The listing builds one solid part. Answer for the finished solid, in the listing's coordinates (mm). A direction names the side the tool comes from. Coordinates: 2 decimals unless noted, no trailing zeros. Order: outer loops, then holes, each group sorted by start corner. A loop starts at its lowest first (then second) coordinate and runs counter-clockwise, first axis right, second up. Notation, with made-up numbers: (26, 82.5) - (55, 82.5) arc R16 cw to (55, 106.5) - close; hole circle Ø3 at (-4.75, 25.25). An arc over 180 degrees is marked (long way). One line per item, written item: value. Start each with the question number.
```python
from build123d import *

# Parameters (mm, degrees)
SKETCH1_W           = 10
SKETCH1_H           = 10
SKETCH1_R           = 1.6
BOSS_EXTRUDE1_DEPTH = 0.5
SKETCH4_W           = 10
SKETCH4_H           = 10
SKETCH4_W_2         = 9
SKETCH4_H_2         = 9
BOSS_EXTRUDE2_DEPTH = 9
SKETCH5_W           = 10
SKETCH5_H           = 10
SKETCH5_R           = 3
BOSS_EXTRUDE3_DEPTH = 0.5
SKETCH6_R           = 3
CUT_EXTRUDE1_DEPTH  = 0.5
SKETCH7_R           = 3
CUT_EXTRUDE2_DEPTH  = 0.5
SKETCH8_R           = 1.6
CUT_EXTRUDE3_DEPTH  = 0.5
SKETCH9_R           = 1.6
CUT_EXTRUDE4_DEPTH  = 0.5
FILLET5_R           = 0.5


with BuildPart() as part:
    # Sketch1 → Boss-Extrude1 (new body)
    with BuildSketch(Plane(origin=(0, 0, 0), x_dir=(1, 0, 0), z_dir=(0, 1, 0))):
        with Locations((5, 5)):
            Rectangle(SKETCH1_W, SKETCH1_H)
        with Locations(Location((5, 5, 0), (0, 0, 270))):
            Circle(SKETCH1_R, mode=Mode.SUBTRACT)
    extrude(amount=BOSS_EXTRUDE1_DEPTH)

    # Sketch4 → Boss-Extrude2 (add)
    with BuildSketch(Plane(origin=(0, 0.5, 0), x_dir=(1, 0, 0), z_dir=(0, 1, 0))):
        with Locations((5, 5)):
            Rectangle(SKETCH4_W, SKETCH4_H)
        with Locations((5, 5)):
            Rectangle(SKETCH4_W_2, SKETCH4_H_2, mode=Mode.SUBTRACT)
    extrude(amount=BOSS_EXTRUDE2_DEPTH)

    # Sketch5 → Boss-Extrude3 (add)
    with BuildSketch(Plane(origin=(0, 9.5, 0), x_dir=(1, 0, 0), z_dir=(0, 1, 0))):
        with Locations((5, 5)):
            Rectangle(SKETCH5_W, SKETCH5_H)
        with Locations(Location((5, 5, 0), (0, 0, 270))):
            Circle(SKETCH5_R, mode=Mode.SUBTRACT)
    extrude(amount=BOSS_EXTRUDE3_DEPTH)

    # Sketch6 → Cut-Extrude1 (cut)
    with BuildSketch(Plane(origin=(10, 0, 0), x_dir=(0, 0, -1), z_dir=(1, 0, 0))):
        with Locations((5, 5)):
            Circle(SKETCH6_R)
    extrude(amount=-CUT_EXTRUDE1_DEPTH, mode=Mode.SUBTRACT)

    # Sketch7 → Cut-Extrude2 (cut)
    with BuildSketch(Plane.XY):
        with Locations((5, 5)):
            Circle(SKETCH7_R)
    extrude(amount=-CUT_EXTRUDE2_DEPTH, mode=Mode.SUBTRACT)

    # Sketch8 → Cut-Extrude3 (cut)
    with BuildSketch(Plane.ZY):
        with Locations((-5, 5)):
            Circle(SKETCH8_R)
    extrude(amount=-CUT_EXTRUDE3_DEPTH, mode=Mode.SUBTRACT)

    # Sketch9 → Cut-Extrude4 (cut)
    with BuildSketch(Plane(origin=(0, 0, -10), x_dir=(-1, 0, 0), z_dir=(0, 0, -1))):
        with Locations((-5, 5)):
            Circle(SKETCH9_R)
    extrude(amount=-CUT_EXTRUDE4_DEPTH, mode=Mode.SUBTRACT)

    # Fillet5
    fillet5_edges = [part.edges().sort_by_distance(p)[0] for p in [
        (0, 10, -5),
        (5, 10, 0),
        (10, 10, -5),
        (5, 10, -10),
        (5, 0, -10),
        (10, 0, -5),
        (5, 0, 0),
        (0, 0, -5),
        (0, 5, -10),
        (10, 5, -10),
        (10, 5, 0),
        (0, 5, 0),
    ]]
    fillet(fillet5_edges, radius=FILLET5_R)


solid = part.part
```
(1) The part is cut by section C-C on x = 6. Determine the outline of the cut face in (y, z).
(2) The part is cut by section A-A on y = 1.25. Determine the outline of the cut face in (x, z), plus the area to 3 significant figures.
(3) For a pull along Z with two mould halves and no side action, classify faces 1 (the face through (2.338, 9.746, -3.616)), 2 (the face through (5, 0, -3)), 3 (the face through (5, 7, -10)) as pulls with the +Z half, pulls with the -Z half, needs draft (parallel to the pull), parting line crosses it, or undercut.
(4) Consider probe 1 along Y at (x, z) = (7.5, -7.75); probe 2 along Z at (x, y) = (7.75, 7). Determine where each line is inside the solid, lowest interval first.
(5) The part is cut by section D-D on y = 6.75. Determine the outline of the cut face in (x, z).
(6) The part is cut by section B-B on z = -5. Determine the outline of the cut face in (x, y), plus the area to 3 significant figures.
(7) Flat-ended cylindrical pins translate along their axes: pin 1 Ø1.9 at (y, z) = (5, -5) entering from -X; pin 2 Ø4.5 at (y, z) = (5.5, -7) entering from +X; pin 3 Ø4 at (x, z) = (5, -5) entering from +Y. Find the tip coordinate at first contact, or state that the pin passes through.
(8) For faces 4 (the face through (4.35, 2.07, -0.25)), 5 (the face through (9.75, 2.07, -4.35)), 6 (the face through (5, 7, -9.5)), determine the directions among +Z, -Z, +X, -X, +Y, -Y from which every point of the face is accessible in a straight line to the end or side of a thin tool.
Completed:
1. outline: (0, -9.5) arc R0.5 ccw to (0.5, -10) - (3.75, -10) - (3.75, -9.5) - (0.5, -9.5) - (0.5, -6.25) - (0, -6.25) - close; (0, -3.75) - (0.5, -3.75) - (0.5, -0.5) - (2.17, -0.5) - (2.17, 0) - (0.5, 0) arc R0.5 ccw to (0, -0.5) - close; (6.25, -10) - (9.5, -10) arc R0.5 ccw to (10, -9.5) - (10, -7.83) - (9.5, -7.83) - (9.5, -9.5) - (6.25, -9.5) - close; (7.83, -0.5) - (9.5, -0.5) - (9.5, -2.17) - (10, -2.17) - (10, -0.5) arc R0.5 ccw to (9.5, 0) - (7.83, 0) - close
2. outline: (0, -9.5) arc R0.5 ccw to (0.5, -10) - (9.5, -10) arc R0.5 ccw to (10, -9.5) - (10, -0.5) arc R0.5 ccw to (9.5, 0) - (0.5, 0) arc R0.5 ccw to (0, -0.5) - close; hole (0.5, -9.5) - (9.5, -9.5) - (9.5, -0.5) - (0.5, -0.5) - close
2. area: 18.8 mm2
3. face 1: undercut
3. face 2: needs draft
3. face 3: pulls with the -Z half
4. probe 1: y = 0 to 0.5, 9.5 to 10
4. probe 2: z = -10 to -9.5, -0.5 to 0
5. outline: (0, -9.5) arc R0.5 ccw to (0.5, -10) - (9.5, -10) arc R0.5 ccw to (10, -9.5) - (10, -7.44) - (9.5, -7.44) - (9.5, -9.5) - (0.5, -9.5) - (0.5, -0.5) - (2.56, -0.5) - (2.56, 0) - (0.5, 0) arc R0.5 ccw to (0, -0.5) - close; (7.44, -0.5) - (9.5, -0.5) - (9.5, -2.56) - (10, -2.56) - (10, -0.5) arc R0.5 ccw to (9.5, 0) - (7.44, 0) - close
6. outline: (0, 0.5) arc R0.5 ccw to (0.5, 0) - (3.4, 0) - (3.4, 0.5) - (0.5, 0.5) - (0.5, 3.4) - (0, 3.4) - close; (0, 6.6) - (0.5, 6.6) - (0.5, 9.5) - (2, 9.5) - (2, 10) - (0.5, 10) arc R0.5 ccw to (0, 9.5) - close; (6.6, 0) - (9.5, 0) arc R0.5 ccw to (10, 0.5) - (10, 2) - (9.5, 2) - (9.5, 0.5) - (6.6, 0.5) - close; (8, 9.5) - (9.5, 9.5) - (9.5, 8) - (10, 8) - (10, 9.5) arc R0.5 ccw to (9.5, 10) - (8, 10) - close
6. area: 9.59 mm2
7. pin 1: passes through
7. pin 2: stops at x = 10
7. pin 3: stops at y = 0.5
8. face 4: +Z
8. face 5: +X
8. face 6: none
